Work out the finished part from the listing and answer in its coordinate system (mm). A direction names the side the tool comes from. Give positions to 0.01 mm unless a question says otherwise; leave off trailing zeros. Loops run counter-clockwise (first coordinate to the right, second up) from the corner with the lowest first, then second, coordinate; pieces in that order, holes last. Notation, with made-up numbers: M -1,68 L 39,68 A14 ccw 39,84 Z; hole C 31.25,39.25 d3. An arc over 180 degrees is marked long. Answer as a JSON object with one key per item and string values. Group by question number.
```python
from build123d import *

# Parameters (mm, degrees)
SKETCH2_R           = 1.5
BOSS_EXTRUDE1_DEPTH = 16
CHAMFER1_SIZE       = 0.3
CUT_EXTRUDE1_DEPTH  = 1.2
SKETCH8_R           = 1.204700538
CUT_EXTRUDE2_DEPTH  = 1
CUT_EXTRUDE2_DRAFT  = -45


with BuildPart() as part:
    # Sketch2 → Boss-Extrude1 (new body)
    with BuildSketch(Plane(origin=(0, 0, 0), x_dir=(0, 0, -1), z_dir=(1, 0, 0))):
        Circle(SKETCH2_R)
    extrude(amount=-BOSS_EXTRUDE1_DEPTH)

    # Chamfer1
    chamfer1_edges = [part.edges().sort_by_distance(p)[0] for p in [
        (0, 0, 1.5),
    ]]
    chamfer(chamfer1_edges, length=CHAMFER1_SIZE)

    # Sketch6 → Revolve1 (revolve)
    with BuildSketch(Plane.XY):
        with BuildLine():
            Line((-17.65, 0), (-17.65, 1.5))
            ThreePointArc((-17.65, 1.5), (-17.055944823, 2.284868705), (-16.25, 2.85))
            Line((-16.25, 2.85), (-16, 2.85))
            Line((-16, 2.85), (-16, 0))
            Line((-16, 0), (-17.65, 0))
        make_face()
    revolve(axis=Axis((-16, 0, 0), (1, 0, 0)))

    # Sketch7 → Cut-Extrude1 (cut)
    with BuildSketch(Plane.ZY.offset(17.65)):
        Polygon((0, 1.154700538), (-1, 0.577350269), (-1, -0.577350269), (0, -1.154700538), (1, -0.577350269), (1, 0.577350269), align=None)
    extrude(amount=-CUT_EXTRUDE1_DEPTH, mode=Mode.SUBTRACT)


with BuildPart() as cut_extrude2_tool:
    # Sketch8 → Cut-Extrude2 (with draft: the straight prism first)
    with BuildSketch(Plane.ZY.offset(17.65)):
        Circle(SKETCH8_R)
    extrude(amount=-CUT_EXTRUDE2_DEPTH)
    # Cut-Extrude2: the draft: its side faces are tilted about the plane it starts from
    cut_extrude2_sides = [cut_extrude2_tool.faces().sort_by_distance(p)[0] for p in [
        (-17.15, 0, -1.204700538),
    ]]
    draft(cut_extrude2_sides, Plane.ZY.offset(17.65), CUT_EXTRUDE2_DRAFT)


with BuildPart() as part_1:
    add(part.part)

    # Cut-Extrude2: cut by cut_extrude2_tool
    add(cut_extrude2_tool.part, mode=Mode.SUBTRACT)


solid = part_1.part
```
Item 1: A cutting plane is placed at D-D (y = 1.8). Determine the outline of the cut face in (x, z).
Item 2: Find the intervals of material crossed by probe 1 along X at (y, z) = (-0.9, -0.1); probe 2 along Z at (x, y) = (-3.75, -0.9); probe 3 along Z at (x, y) = (-5.5, -0.1), in increasing order. Write a range as [from, to].
Item 3: A cutting plane is placed at B-B (x = -9.5). Determine the outline of the cut face in (y, z), and give its area (3 significant figures).
Item 4: A cutting plane is placed at C-C (z = -2.05). Determine the outline of the cut face in (x, y), and give its area (3 significant figures).
Item 5: A tool of negligible diameter and unlimited length cuts with its end or side. For faces 1 (the flat face through (-17.03, 0.87, -0.49)), 2 (the flat face through (-16, 1.2, -1.2)), from which of +Z, -Z, +X, -X, +Y, -Y can it reach the whole face along a straight path? Write none if from no direction.
Item 6: For a pull along Z with two mould halves and no side action, classify faces 3 (the cylindrical face through (-8.04, 0.07, 1.5)), 4 (the flat face through (0, 0, 0)), 5 (the flat face through (-17.03, -0.87, 0.49)) as pulls with the +Z half, pulls with the -Z half, needs draft (parallel to the pull), parting line crosses it, or undercut.
Item 7: Given pin 1 Ø0.6 at (x, y) = (-17, 0) entering from +Z; pin 2 Ø1 at (x, z) = (-2.5, 0.5) entering from +Y; pin 3 Ø1.3 at (x, y) = (-17, 0) entering from -Z, each flat-ended and moving along its own axis, determine where each tip first touches the part or whether it passes through.
Item 8: A cutting plane is placed at A-A (y = 0). Determine the outline of the cut face in (x, z).
The answers:
{
 "1": {"outline": "M -16.25,-2.21 L -16,-2.21 L -16,2.21 L -16.25,2.21 A2.61 ccw Z"},
 "2": {"probe 1": "x = [-16.45, 0]", "probe 2": "z = [-1.2, 1.2]", "probe 3": "z = [-1.5, 1.5]"},
 "3": {"outline": "C 0,0 d3", "area": "7.07 mm^2"},
 "4": {"outline": "M -16.25,-1.98 L -16,-1.98 L -16,1.98 L -16.25,1.98 A2.42 ccw Z", "area": "3.84 mm^2"},
 "5": {"face 1": "-X", "face 2": "+X"},
 "6": {"face 3": "parting line crosses it", "face 4": "needs draft", "face 5": "undercut"},
 "7": {"pin 1": "stops at z = 2.58", "pin 2": "stops at y = 1.5", "pin 3": "stops at z = -2.8"},
 "8": {"outline": "M -17.65,-1.5 A3.17 ccw -16.25,-2.85 L -16,-2.85 L -16,-1.5 L -0.3,-1.5 L 0,-1.2 L 0,1.2 L -0.3,1.5 L -16,1.5 L -16,2.85 L -16.25,2.85 A3.17 ccw -17.65,1.5 L -17.65,1.2 L -17.45,1 L -16.45,1 L -16.45,-1 L -17.45,-1 L -17.65,-1.2 Z"}
}
